For this review, take the finished solid that the model builds, in its own axes (mm). A direction names the side the tool comes from. Round coordinates to 2 decimals unless told otherwise and drop trailing zeros. Order: outer loops, then holes, each group sorted by start corner. A loop starts at its lowest first (then second) coordinate and runs counter-clockwise, first axis right, second up. Notation, with made-up numbers: (42, 43) -> (85, 43) arc R3 cw to (85, 47) -> close; hole circle Ø11 at (42, 42). An arc over 180 degrees is marked (long way). Use a Markdown table: item, result. Add a question column.
1) Clearance check with flat-ended pins moving along their axes: P1, Ø1.5, axis at y = 2, z = -7.5, coming from the +X side; P2, Ø1.5, axis at x = -1.5, y = 2.5, coming from the -Z side. State where each tip first meets the part, or that it passes through.
2) Wall thickness on line 1 along X through (y, z) = (7.85, 0) (1 decimal); line 2 along Z through (x, y) = (-1, 5.5); line 3 along Z through (x, y) = (5.5, 4.5): over which ranges is each line inside the solid? List them lowest first. Write a range as [from, to].
3) Draft analysis for pull direction X (two halves, no side actions). For faces 5 (the face through (0.628, 4.455, -14.274)), 6 (the face through (-2.72, 3.91, -5.74)), 7 (the face through (6.2, 7.925, -10.3)), state which applies: pulls with the +X half, pulls with the -X half, needs draft (parallel to the pull), parting line crosses it, or undercut.
4) Consider section A-A (y = 5.5). State the section outline as (x, z) points (1 decimal).
5) Machinability: for faces 1 (the face through (0, 0.152, -10)), 2 (the face through (-12.194, 1.575, 7.735)), 3 (the face through (12, 0, 2)), 4 (the face through (6.33, 3.91, 0.51)), which of the approach directions +Z, -Z, +X, -X, +Y, -Y give a long, thin tool a straight path to every point of the face, cutting with its end or side? Answer none if there is none.
```python
from build123d import *

# Parameters (mm, degrees)
SKETCH1_R                = 9.525
BOSS_EXTRUDE1_DEPTH      = 7.9248
SKETCH2_R                = 11.67450685
SKETCH2_R_2              = 9.525
BOSS_EXTRUDE2_DEPTH      = 3.81
BOSS_EXTRUDE2_DEPTH_BACK = 3.81
SKETCH3_R                = 14.2875
SKETCH3_R_2              = 11.67450685
BOSS_EXTRUDE4_DEPTH      = 7.9248
SKETCH4_R                = 15.56004
SKETCH4_R_2              = 14.2875
BOSS_EXTRUDE5_DEPTH      = 1.5748
FILLET1_R                = 0.508


with BuildPart() as part:
    # Sketch1 → Boss-Extrude1 (new body)
    with BuildSketch(Plane(origin=(0, 0, 0), x_dir=(1, 0, 0), z_dir=(0, 1, 0))):
        with Locations(Location((0, 0, 0), (0, 0, 270))):
            Circle(SKETCH1_R)
        Polygon((6.069005203, -4.114669997), (6.597911347, 3.198577683), (0.528906144, 7.31324768), (-6.069005203, 4.114669997), (-6.597911347, -3.198577683), (-0.528906144, -7.31324768), align=None, mode=Mode.SUBTRACT)
    extrude(amount=BOSS_EXTRUDE1_DEPTH)



with BuildPart() as body_2:
    # Sketch2 → Boss-Extrude2 (new, two sides)
    with BuildSketch(Plane(origin=(0, 3.9624, 0), x_dir=(1, 0, 0), z_dir=(0, 1, 0))) as boss_extrude2_sk:
        with Locations(Location((0, 0, 0), (0, 0, 270))):
            Circle(SKETCH2_R)
        with Locations(Location((0, 0, 0), (0, 0, 270))):
            Circle(SKETCH2_R_2, mode=Mode.SUBTRACT)
    extrude(amount=BOSS_EXTRUDE2_DEPTH)
    extrude(boss_extrude2_sk.sketch, amount=-BOSS_EXTRUDE2_DEPTH_BACK)


with BuildPart() as part_1:
    add(part.part)

    add(body_2.part)  # Boss-Extrude4 merges body 2
    # Sketch3 → Boss-Extrude4 (add)
    with BuildSketch(Plane(origin=(0, 0, 0), x_dir=(1, 0, 0), z_dir=(0, 1, 0))):
        with Locations(Location((0, 0, 0), (0, 0, 270))):
            Circle(SKETCH3_R)
        with Locations(Location((0, 0, 0), (0, 0, 270))):
            Circle(SKETCH3_R_2, mode=Mode.SUBTRACT)
    extrude(amount=BOSS_EXTRUDE4_DEPTH)

    # Sketch4 → Boss-Extrude5 (add)
    with BuildSketch(Plane(origin=(0, 0, 0), x_dir=(1, 0, 0), z_dir=(0, 1, 0))):
        with Locations(Location((0, 0, 0), (0, 0, 270))):
            Circle(SKETCH4_R)
        with Locations(Location((0, 0, 0), (0, 0, 270))):
            Circle(SKETCH4_R_2, mode=Mode.SUBTRACT)
    extrude(amount=BOSS_EXTRUDE5_DEPTH)

    # Fillet1
    fillet1_edges = [part_1.edges().sort_by_distance(p)[0] for p in [
        (0, 7.9248, -14.2875),
        (0, 1.5748, -15.56004),
    ]]
    fillet(fillet1_edges, radius=FILLET1_R)


solid = part_1.part
```
Results list:
| question | item | result |
|---|---|---|
| 1 | P1 | x = 13.74 |
| 1 | P2 | z = -14.27 |
| 2 | line 1 | [-14, -11.7], [-9.5, -6.4], [6.4, 9.5], [11.7, 14] |
| 2 | line 2 | [-14.25, -6.57], [6.99, 14.25] |
| 2 | line 3 | [-13.19, -3.94], [4.39, 13.19] |
| 3 | face 5 | parting line crosses it |
| 3 | face 6 | undercut |
| 3 | face 7 | needs draft |
| 4 | outline | circle Ø28.6 at (0, 0); hole (-6.6, 3.2) -> (-6.1, -4.1) -> (0.5, -7.3) -> (6.6, -3.2) -> (6.1, 4.1) -> (-0.5, 7.3) -> close |
| 5 | face 1 | -Y |
| 5 | face 2 | +Y |
| 5 | face 3 | +Z, -Z, +X, -X, -Y |
| 5 | face 4 | +Y, -Y |
